Build history of the part. All positions in model axes, mm. Give positions to 0.01 mm unless a question says otherwise; leave off trailing zeros. Write each loop counter-clockwise with the first axis right and the second up, starting at its lowest first coordinate (ties: lowest second). Pieces come first, ordered by that corner, then holes. Notation, with made-up numbers: (56.25, 24) -> (60.25, 24) arc R19 cw to (60.25, 44) -> close; hole circle Ø8 at (84, 89.5). An arc over 180 degrees is marked (long way). Put each result on its own line as item: value.
from build123d import *

# Parameters (mm, degrees)
SKETCH1_R           = 95.885
SKETCH1_R_2         = 6.35
BOSS_EXTRUDE1_DEPTH = 4.7625


with BuildPart() as part:
    # Sketch1 → Boss-Extrude1 (new body)
    with BuildSketch(Plane(origin=(0, 0, 0), x_dir=(1, 0, 0), z_dir=(0, 1, 0))):
        with BuildLine():
            Line((127, -127), (-127, -127))
            Line((-127, -127), (-127, 0))
            ThreePointArc((-127, 0), (-89.802561208, 89.802561213), (7e-09, 127))
            ThreePointArc((7e-09, 127), (88.687133546, 90.920457479), (127, 3.175))
            Line((127, 3.175), (127, -127))
        make_face()
        Circle(SKETCH1_R, mode=Mode.SUBTRACT)
        with Locations((-108.072773191, -37.212440054)):
            Circle(SKETCH1_R_2, mode=Mode.SUBTRACT)
        with Locations((21.809468172, 112.199987068)):
            Circle(SKETCH1_R_2, mode=Mode.SUBTRACT)
        with Locations((86.263305019, -74.987547014)):
            Circle(SKETCH1_R_2, mode=Mode.SUBTRACT)
        with Locations((-63.5, -114.3)):
            Circle(SKETCH1_R_2, mode=Mode.SUBTRACT)
        with Locations((63.5, -114.3)):
            Circle(SKETCH1_R_2, mode=Mode.SUBTRACT)
    extrude(amount=BOSS_EXTRUDE1_DEPTH)


solid = part.part
1) Slice it at D-D (z = -20.5). Write the cut outline in (x, y).
Filled sheet:
outline: (-125.33, 0) -> (-93.67, 0) -> (-93.67, 4.76) -> (-125.33, 4.76) -> close; (93.67, 0) -> (125.37, 0) -> (125.37, 4.76) -> (93.67, 4.76) -> close
2) Pin check, flat tip, straight feed: pin 1 (10 mm diameter, centred on x = -108.07, z = 37.21, fed in from -Y). Stop position of the tip, or through.
Filled sheet:
pin 1: through
3) Pull direction Z, two halves, no side cores. Call faces 1 (the flat face through (-55, 4.762, 83)), 2 (the cylindrical face through (87.7, 2.35, -91.87)), 3 (the cylindrical face through (20.43, 2.35, -106)): released by +Z, released by -Z, zero draft, split by the parting line, or undercut.
Filled sheet:
face 1: zero draft
face 2: released by -Z
face 3: undercut
4) Slice it at B-B (x = -61). Write the cut outline in (y, z).
Filled sheet:
outline: (0, -111.39) -> (4.76, -111.39) -> (4.76, -73.98) -> (0, -73.98) -> close; (0, 73.98) -> (4.76, 73.98) -> (4.76, 108.46) -> (0, 108.46) -> close; (0, 120.14) -> (4.76, 120.14) -> (4.76, 127) -> (0, 127) -> close
5) Slice it at A-A (z = 114.3). Write the cut outline in (x, y), plus the area to 3 significant figures.
Filled sheet:
outline: (-127, 0) -> (-69.85, 0) -> (-69.85, 4.76) -> (-127, 4.76) -> close; (-57.15, 0) -> (57.15, 0) -> (57.15, 4.76) -> (-57.15, 4.76) -> close; (69.85, 0) -> (127, 0) -> (127, 4.76) -> (69.85, 4.76) -> close
area: 1,090 mm2
6) Slice it at C-C (y = 2.5). Write the cut outline in (x, z) (3 decimals), plus the area to 3 significant figures.
Filled sheet:
outline: (-127, 0) arc R127 ccw to (0, -127) arc R127.041 ccw to (127, -3.175) -> (127, 127) -> (-127, 127) -> close; hole circle Ø12.7 at (-108.073, 37.212); hole circle Ø191.77 at (0, 0); hole circle Ø12.7 at (-63.5, 114.3); hole circle Ø12.7 at (21.809, -112.2); hole circle Ø12.7 at (63.5, 114.3); hole circle Ø12.7 at (86.263, 74.988)
area: 28,100 mm2
7) Wall check: L1, parallel to X at y = 0.45, z = 2; L2, parallel to X at y = 3.05, z = 114.3; L3, parallel to Z at x = 63.5, y = 1.2. Give the ranges that are in metal, low to high.
Filled sheet:
L1: -127 to -95.86, 95.86 to 127
L2: -127 to -69.85, -57.15 to 57.15, 69.85 to 127
L3: -109.99 to -71.84, 71.84 to 107.95, 120.65 to 127
